Geometry check sheet. Reference: the model listing, model coordinates, mm. Face numbers are marked on the shaded views. A direction names the side the tool comes from. Round coordinates to 2 decimals unless told otherwise and drop trailing zeros. Order: outer loops, then holes, each group sorted by start corner. A loop starts at its lowest first (then second) coordinate and runs counter-clockwise, first axis right, second up. Notation, with made-up numbers: (-3, -24) -> (48, -24) arc R16 ccw to (48, -20) -> close; hole circle Ø11 at (46, 62.5). An arc over 180 degrees is marked (long way). Use a Markdown table: item, result. Add a question column.
Item 1: Sectioned sample at C-C, the plane y = -19. Record the cut outline in (x, z).
Item 2: Gauge pin test, flat ends, axial feed: pin 1 Ø1.2 at (x, z) = (-6.5, 41.25) entering from -Y; pin 2 Ø12 at (x, y) = (-3.5, 1) entering from +Z; pin 3 Ø1 at (x, z) = (-3, 53.5) entering from -Y. Record the tip position at first contact, or that the pin passes through.
Item 3: Sectioned sample at B-B, the plane y = -10.5. Record the cut outline in (x, z), and give its area (3 significant figures).
Item 4: Sectioned sample at A-A, the plane z = 34.5. Record the cut outline in (x, y), and give its area (3 significant figures).
Item 5: Set-up check for the marked faces 1 and 2: record each of +Z, -Z, +X, -X, +Y, -Y from which the full face is reachable in a straight line by a thin tool's end or side.
Item 6: Material ranges on probe 1 along Z at (x, y) = (9, 18.5); probe 2 along X at (y, z) = (18.85, 39.75); probe 3 along X at (y, z) = (20.4, 38.25), recorded low to high. Write a range as [from, to].
from build123d import *

# Parameters (mm, degrees)
SKETCH1_W           = 45
SKETCH1_H           = 45
SKETCH1_R           = 1
BOSS_EXTRUDE1_DEPTH = 5
SKETCH2_W           = 45
SKETCH2_H           = 5
BOSS_EXTRUDE2_DEPTH = 60
SKETCH3_R           = 1
CUT_EXTRUDE1_DEPTH  = 5


with BuildPart() as part:
    # Sketch1 → Boss-Extrude1 (new body)
    with BuildSketch(Plane.XY):
        Rectangle(SKETCH1_W, SKETCH1_H)
        with Locations((0, -13.5)):
            Circle(SKETCH1_R, mode=Mode.SUBTRACT)
        with Locations((0, -10.5)):
            Circle(SKETCH1_R, mode=Mode.SUBTRACT)
        with Locations((0, -7.5)):
            Circle(SKETCH1_R, mode=Mode.SUBTRACT)
        with Locations((-11.691342951, -6.75)):
            Circle(SKETCH1_R, mode=Mode.SUBTRACT)
        with Locations((-9.09326674, -5.25)):
            Circle(SKETCH1_R, mode=Mode.SUBTRACT)
        with Locations((-6.495190528, -3.75)):
            Circle(SKETCH1_R, mode=Mode.SUBTRACT)
        with Locations((-11.691342951, 6.75)):
            Circle(SKETCH1_R, mode=Mode.SUBTRACT)
        with Locations((-9.09326674, 5.25)):
            Circle(SKETCH1_R, mode=Mode.SUBTRACT)
        with Locations((-6.495190528, 3.75)):
            Circle(SKETCH1_R, mode=Mode.SUBTRACT)
        with Locations((0, 13.5)):
            Circle(SKETCH1_R, mode=Mode.SUBTRACT)
        with Locations((0, 10.5)):
            Circle(SKETCH1_R, mode=Mode.SUBTRACT)
        with Locations((0, 7.5)):
            Circle(SKETCH1_R, mode=Mode.SUBTRACT)
        with Locations((11.691342951, 6.75)):
            Circle(SKETCH1_R, mode=Mode.SUBTRACT)
        with Locations((9.09326674, 5.25)):
            Circle(SKETCH1_R, mode=Mode.SUBTRACT)
        with Locations((6.495190528, 3.75)):
            Circle(SKETCH1_R, mode=Mode.SUBTRACT)
        with Locations((11.691342951, -6.75)):
            Circle(SKETCH1_R, mode=Mode.SUBTRACT)
        with Locations((9.09326674, -5.25)):
            Circle(SKETCH1_R, mode=Mode.SUBTRACT)
        with Locations((6.495190528, -3.75)):
            Circle(SKETCH1_R, mode=Mode.SUBTRACT)
    extrude(amount=BOSS_EXTRUDE1_DEPTH)

    # Sketch2 → Boss-Extrude2 (add)
    with BuildSketch(Plane.XY.offset(5)):
        with Locations((0, 20)):
            Rectangle(SKETCH2_W, SKETCH2_H)
    extrude(amount=BOSS_EXTRUDE2_DEPTH)

    # Sketch3 → Cut-Extrude1 (cut)
    with BuildSketch(Plane(origin=(-5, 17.5, 0), x_dir=(0, 0, -1), z_dir=(0, 1, 0))):
        with Locations((-58.5, -5)):
            Circle(SKETCH3_R)
        with Locations((-55.5, -5)):
            Circle(SKETCH3_R)
        with Locations((-52.5, -5)):
            Circle(SKETCH3_R)
        with Locations((-51.75, 6.691342951)):
            Circle(SKETCH3_R)
        with Locations((-50.25, 4.09326674)):
            Circle(SKETCH3_R)
        with Locations((-48.75, 1.495190528)):
            Circle(SKETCH3_R)
        with Locations((-38.25, 6.691342951)):
            Circle(SKETCH3_R)
        with Locations((-39.75, 4.09326674)):
            Circle(SKETCH3_R)
        with Locations((-41.25, 1.495190528)):
            Circle(SKETCH3_R)
        with Locations((-31.5, -5)):
            Circle(SKETCH3_R)
        with Locations((-34.5, -5)):
            Circle(SKETCH3_R)
        with Locations((-37.5, -5)):
            Circle(SKETCH3_R)
        with Locations((-38.25, -16.691342951)):
            Circle(SKETCH3_R)
        with Locations((-39.75, -14.09326674)):
            Circle(SKETCH3_R)
        with Locations((-41.25, -11.495190528)):
            Circle(SKETCH3_R)
        with Locations((-51.75, -16.691342951)):
            Circle(SKETCH3_R)
        with Locations((-50.25, -14.09326674)):
            Circle(SKETCH3_R)
        with Locations((-48.75, -11.495190528)):
            Circle(SKETCH3_R)
    extrude(amount=CUT_EXTRUDE1_DEPTH, mode=Mode.SUBTRACT)


solid = part.part
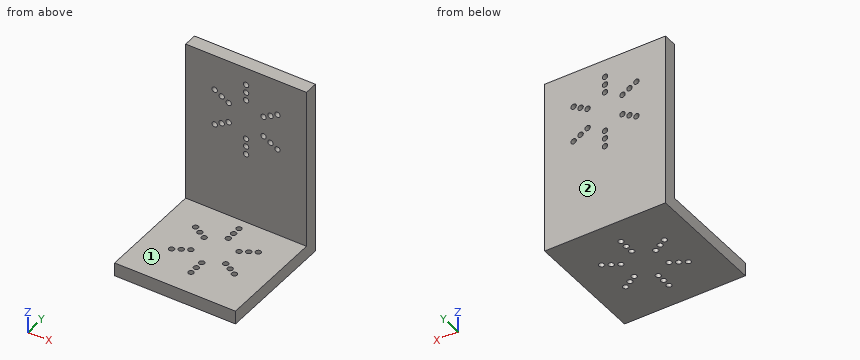
Found:
| question | item | result |
|---|---|---|
| 1 | outline | (-22.5, 0) -> (22.5, 0) -> (22.5, 5) -> (-22.5, 5) -> close |
| 2 | pin 1 | passes through |
| 2 | pin 2 | stops at z = 5 |
| 2 | pin 3 | stops at y = 17.5 |
| 3 | outline | (-22.5, 0) -> (-1, 0) -> (-1, 5) -> (-22.5, 5) -> close; (1, 0) -> (22.5, 0) -> (22.5, 5) -> (1, 5) -> close |
| 3 | area | 215 mm2 |
| 4 | outline | (-22.5, 17.5) -> (-1, 17.5) -> (-1, 22.5) -> (-22.5, 22.5) -> close; (1, 17.5) -> (22.5, 17.5) -> (22.5, 22.5) -> (1, 22.5) -> close |
| 4 | area | 215 mm2 |
| 5 | face 1 | +Z, +X, -X, -Y |
| 5 | face 2 | +Z, -Z, +X, -X, +Y |
| 6 | probe 1 | z = [0, 38.75], [40.75, 49.25], [51.25, 65] |
| 6 | probe 2 | x = [-22.5, -10.09], [-8.09, 8.09], [10.09, 22.5] |
| 6 | probe 3 | x = [-22.5, -12.69], [-10.69, -0.66], [0.66, 10.69], [12.69, 22.5] |
